Here's how the part is built. I have some questions about the finished solid (model axes, mm). A direction names the side the tool comes from. Round coordinates to 2 decimals unless told otherwise and drop trailing zeros. Loops run counter-clockwise (first coordinate to the right, second up) from the corner with the lowest first, then second, coordinate; pieces in that order, holes last. Notation, with made-up numbers: M 26,61 L 59,61 A14 cw 59,80 Z; hole C 39,46 d6. An arc over 180 degrees is marked long. Write each question's results on one line, items separated by ' | '. Start each with the question number.
```python
from build123d import *

# Parameters (mm, degrees)
BOSS_EXTRUDE1_DEPTH = 58.6
SKETCH2_R           = 1.6
CUT_EXTRUDE1_DEPTH  = 58.6


with BuildPart() as part:
    # Sketch1 → Boss-Extrude1 (new body)
    with BuildSketch(Plane.XY):
        with BuildLine():
            Line((-23.65, 6), (-14.4, 6))
            ThreePointArc((-14.4, 6), (0, 15.6), (14.4, 6))
            Line((14.4, 6), (23.65, 6))
            Line((23.65, 6), (23.65, 2))
            Line((23.65, 2), (12.440257232, 2))
            ThreePointArc((12.440257232, 2), (0, 12.6), (-12.440257232, 2))
            Line((-12.440257232, 2), (-23.65, 2))
            Line((-23.65, 2), (-23.65, 6))
        make_face()
    extrude(amount=BOSS_EXTRUDE1_DEPTH)

    # Sketch2 → Cut-Extrude1 (cut)
    with BuildSketch(Plane(origin=(0, 6, 0), x_dir=(1, 0, 0), z_dir=(0, 1, 0))):
        with Locations((18.65, -5)):
            Circle(SKETCH2_R)
        with Locations((18.65, -53.6)):
            Circle(SKETCH2_R)
        with Locations((-18.65, -53.6)):
            Circle(SKETCH2_R)
        with Locations((-18.65, -5)):
            Circle(SKETCH2_R)
        with Locations((-18.65, -33.6)):
            Circle(SKETCH2_R)
    extrude(amount=-CUT_EXTRUDE1_DEPTH, mode=Mode.SUBTRACT)


solid = part.part
```
1. For pin 1 (10 mm diameter, centred on x = 15.5, z = 29.5, fed in from +Y); pin 2 (5 mm diameter, centred on x = 18.65, z = 53.6, fed in from +Y); pin 3 (3 mm diameter, centred on x = 5, z = 51.5, fed in from +Y), each with a flat end and sliding along its axis, tell me the tip position at first contact or that it passes through.
2. I want a section at B-B on z = 33.6. List the corners of the cut face in (x, y) for me, plus the area to 3 significant figures.
3. I want a section at C-C on y = 4.5. List the corners of the cut face in (x, z) for me.
4. I need wall thicknesses on line 1 along Z through (x, y) = (18.65, 3.9); line 2 along Z through (x, y) = (-18.65, 4.7); line 3 along X through (y, z) = (5.15, 5). Which ranges of each line are inside material? Lowest first, please.
5. Which directions (+Z, -Z, +X, -X, +Y, -Y) give clear straight access to the entire face, cutting with the end or side of a thin tool? Please do faces 5 (the face through (0, 13, 0)), 6 (the face through (-19, 6, 29)), 7 (the face through (19, 6, 29)).
6. I want a section at A-A on x = 18.65. List the corners of the cut face in (y, z) for me.
7. If we mould it in two halves opening along X, with no side actions, what happens to faces 1 (the face through (-19.83, 4.03, 3.92)), 2 (the face through (-0.257, 15.598, 28.89)), 3 (the face through (0.2, 12.6, 28.9)), 4 (the face through (18, 2, 29))? For each: released by +X, released by -X, zero draft, split by the parting line, or undercut.
8. I want a section at D-D on z = 53.6. List the corners of the cut face in (x, y) for me.
Outcome:
1) pin 1: y = 11.54 | pin 2: y = 6 | pin 3: y = 15.2
2) outline: M -23.65,2 L -20.25,2 L -20.25,6 L -23.65,6 Z; M -17.05,2 L -12.44,2 A12.6 cw 12.44,2 L 23.65,2 L 23.65,6 L 14.4,6 A15.6 ccw -14.4,6 L -17.05,6 Z | area: 177 mm2
3) outline: M -23.65,0 L -11.77,0 L -11.77,58.6 L -23.65,58.6 Z; M 11.77,0 L 23.65,0 L 23.65,58.6 L 11.77,58.6 Z; hole C -18.65,5 d3.2; hole C -18.65,33.6 d3.2; hole C -18.65,53.6 d3.2; hole C 18.65,5 d3.2; hole C 18.65,53.6 d3.2
4) line 1: 0 to 3.4, 6.6 to 52, 55.2 to 58.6 | line 2: 0 to 3.4, 6.6 to 32, 35.2 to 52, 55.2 to 58.6 | line 3: -23.65 to -20.25, -17.05 to -11.5, 11.5 to 17.05, 20.25 to 23.65
5) face 5: -Z, +X, -X, +Y, -Y | face 6: +Z, -Z, -X, +Y | face 7: +Z, -Z, +X, +Y
6) outline: M 2,0 L 6,0 L 6,3.4 L 2,3.4 Z; M 2,6.6 L 6,6.6 L 6,52 L 2,52 Z; M 2,55.2 L 6,55.2 L 6,58.6 L 2,58.6 Z
7) face 1: undercut | face 2: split by the parting line | face 3: undercut | face 4: zero draft
8) outline: M -23.65,2 L -20.25,2 L -20.25,6 L -23.65,6 Z; M -17.05,2 L -12.44,2 A12.6 cw 12.44,2 L 17.05,2 L 17.05,6 L 14.4,6 A15.6 ccw -14.4,6 L -17.05,6 Z; M 20.25,2 L 23.65,2 L 23.65,6 L 20.25,6 Z
